Read the model definition and answer for the solid it produces. Units are mm, in the model's axes. A direction names the side the tool comes from. Round coordinates to 2 decimals unless told otherwise and drop trailing zeros. Write each loop counter-clockwise with the first axis right and the second up, starting at its lowest first coordinate (ties: lowest second). Pieces come first, ordered by that corner, then holes. Notation, with made-up numbers: (27, 56.5) -> (32, 56.5) arc R10 cw to (32, 68.5) -> close; hole circle Ø7 at (52, 7.5). An arc over 180 degrees is marked (long way). Return JSON: item names as keys, results as strings.
from build123d import *

# Parameters (mm, degrees)
EKSTR_ZYON_NCE10_DEPTH                = 420
M12_HELISARMAL_I_IN_Z_VANA_MATKAB_1_D = 12.5
M12_HELISARMAL_I_IN_Z_VANA_MATKAB_2_D = 12.25
M10_HELISARMAL_I_IN_Z_VANA_MATKAB_1_D = 10.5
RADYUS1_R                             = 25
RADYUS2_R                             = 25


with BuildPart() as part:
    # Çizim1 → Ekstrüzyon-İnce10 (new body)
    with BuildSketch(Plane.XY):
        with BuildLine():
            Line((-37.044551646, -1.625), (-37.044551646, 40.375))
            ThreePointArc((-37.044551646, 40.375), (-36.751658427, 41.082106781), (-36.044551646, 41.375))
            Line((-36.044551646, 41.375), (3.955448354, 41.375))
            ThreePointArc((3.955448354, 41.375), (4.662555135, 41.082106781), (4.955448354, 40.375))
            Line((4.955448354, 40.375), (4.955448354, -1.625))
            Line((4.955448354, -1.625), (7.955448354, -1.625))
            Line((7.955448354, -1.625), (7.955448354, 40.375))
            ThreePointArc((7.955448354, 40.375), (6.783875479, 43.203427125), (3.955448354, 44.375))
            Line((3.955448354, 44.375), (-36.044551646, 44.375))
            ThreePointArc((-36.044551646, 44.375), (-38.872978771, 43.203427125), (-40.044551646, 40.375))
            Line((-40.044551646, 40.375), (-40.044551646, -1.625))
            Line((-40.044551646, -1.625), (-37.044551646, -1.625))
        make_face()
    extrude(amount=EKSTR_ZYON_NCE10_DEPTH)

    # M12 Helisarmal için Zıvana matkabı1 (through all)
    with Locations(Plane.ZY.offset(40.044551646)):
        with Locations((40, 20.375)):
            Hole(M12_HELISARMAL_I_IN_Z_VANA_MATKAB_1_D / 2)

    # M12 Helisarmal için Zıvana matkabı2 (through all)
    with Locations(Plane.ZY.offset(40.044551646)):
        with Locations((405, 20.375)):
            Hole(M12_HELISARMAL_I_IN_Z_VANA_MATKAB_2_D / 2)

    # M10 Helisarmal için Zıvana matkabı1 (through all)
    with Locations(Plane(origin=(-16.044551646, 44.375, 380), x_dir=(0, 0, 1), z_dir=(0, 1, 0))):
        with Locations((0, 0), (-340, 0)):
            Hole(M10_HELISARMAL_I_IN_Z_VANA_MATKAB_1_D / 2)

    # Radyus1
    radyus1_edges = [part.edges().sort_by_distance(p)[0] for p in [
        (-38.544551646, -1.625, 420),
    ]]
    fillet(radyus1_edges, radius=RADYUS1_R)

    # Radyus2
    radyus2_edges = [part.edges().sort_by_distance(p)[0] for p in [
        (6.455448354, -1.625, 420),
    ]]
    fillet(radyus2_edges, radius=RADYUS2_R)


solid = part.part
Item 1: A tool of negligible diameter and unlimited length cuts with its end or side. For faces 5 (the flat face through (-37.045, 19, 207)), 6 (the flat face through (-16, 44.375, 207)), from which of +Z, -Z, +X, -X, +Y, -Y can it reach the whole face along a straight path? Write none if from no direction.
Worked answers:
{"face 5": "+Z, -Z, -Y", "face 6": "+Z, -Z, +X, -X, +Y"}
Item 2: Straight lines are drawn through the part: L1, parallel to X at y = 16, z = 225; L2, parallel to Y at x = -25, z = 345 (3 decimals); L3, parallel to Y at x = 7.35, z = 40 (3 decimals). For each, find the intervals that lie inside material, in ascending order. Write a range as [from, to].
Worked answers:
{"L1": "x = [-40.04, -37.04], [4.96, 7.96]", "L2": "y = [41.375, 44.375]", "L3": "y = [-1.625, 14.125], [26.625, 42.491]"}
Item 3: Section D-D (x = -32) is taken. Give the vertices of the cut face in (y, z) (3 decimals).
Worked answers:
{"outline": "(41.375, 0) -> (44.375, 0) -> (44.375, 420) -> (41.375, 420) -> close"}
Item 4: Section B-B (y = 36) is taken. Give the vertices of the cut face in (x, z).
Worked answers:
{"outline": "(-40.04, 0) -> (-37.04, 0) -> (-37.04, 420) -> (-40.04, 420) -> close; (4.96, 0) -> (7.96, 0) -> (7.96, 420) -> (4.96, 420) -> close"}
Item 5: Section A-A (z = 380) is taken. Give the vertices of the cut face in (x, y) (3 decimals), then the cut area to 3 significant figures.
Worked answers:
{"outline": "(-40.045, -1.625) -> (-37.045, -1.625) -> (-37.045, 40.375) arc R1 cw to (-36.045, 41.375) -> (-21.295, 41.375) -> (-21.295, 44.375) -> (-36.045, 44.375) arc R4 ccw to (-40.045, 40.375) -> close; (-10.795, 41.375) -> (3.955, 41.375) arc R1 cw to (4.955, 40.375) -> (4.955, -1.625) -> (7.955, -1.625) -> (7.955, 40.375) arc R4 ccw to (3.955, 44.375) -> (-10.795, 44.375) -> close", "area": "364 mm2"}
Item 6: Section C-C (z = 40) is taken. Give the vertices of the cut face in (x, y) (3 decimals), then the cut area to 3 significant figures.
Worked answers:
{"outline": "(-40.045, -1.625) -> (-37.045, -1.625) -> (-37.045, 14.125) -> (-40.045, 14.125) -> close; (-40.045, 26.625) -> (-37.045, 26.625) -> (-37.045, 40.375) arc R1 cw to (-36.045, 41.375) -> (-21.295, 41.375) -> (-21.295, 44.375) -> (-36.045, 44.375) arc R4 ccw to (-40.045, 40.375) -> close; (-10.795, 41.375) -> (3.955, 41.375) arc R1 cw to (4.955, 40.375) -> (4.955, 26.625) -> (7.955, 26.625) -> (7.955, 40.375) arc R4 ccw to (3.955, 44.375) -> (-10.795, 44.375) -> close; (4.955, -1.625) -> (7.955, -1.625) -> (7.955, 14.125) -> (4.955, 14.125) -> close", "area": "289 mm2"}
Item 7: For a pull along Z with two mould halves and no side action, classify faces 1 (the cylindrical face through (6.476, 17.981, 34.227)), 2 (the flat face through (-20, 42, 0)), 3 (the cylindrical face through (6.48, 5.89, 412.87)), 4 (the cylindrical face through (-19.239, 42.854, 44.166)) as released by +Z, released by -Z, zero draft, split by the parting line, or undercut.
Worked answers:
{"face 1": "undercut", "face 2": "released by -Z", "face 3": "released by +Z", "face 4": "undercut"}
Item 8: Flat-ended cylindrical pins translate along their axes: pin 1 (12 mm diameter, centred on x = -16.04, z = 40, fed in from +Y) (3 decimals); pin 2 (6.5 mm diameter, centred on x = -16.04, z = 380, fed in from +Y). Find the tip coordinate at first contact, or state that the pin passes through.
Worked answers:
{"pin 1": "stops at y = 44.375", "pin 2": "passes through"}
